```python
from build123d import *

# Parameters (mm, degrees)
SKETCH1_W                    = 38.1
SKETCH1_H                    = 38.1
SKETCH1_W_2                  = 31.75
SKETCH1_H_2                  = 31.75
BOSS_EXTRUDE1_DEPTH          = 238.125
F_10_0_1935_DIAMETER_HOLE2_D = 4.9149


with BuildPart() as part:
    # Sketch1 → Boss-Extrude1 (new body)
    with BuildSketch(Plane.XY):
        Rectangle(SKETCH1_W, SKETCH1_H)
        Rectangle(SKETCH1_W_2, SKETCH1_H_2, mode=Mode.SUBTRACT)
    extrude(amount=BOSS_EXTRUDE1_DEPTH)

    # #10 (0.1935) Diameter Hole2 (through all)
    with Locations(Plane(origin=(0, 19.05, 0), x_dir=(1, 0, 0), z_dir=(0, 1, 0))):
        with Locations((0, -31.75), (0, -89.958333333), (0, -148.166666667), (0, -206.375)):
            Hole(F_10_0_1935_DIAMETER_HOLE2_D / 2)


solid = part.part
```
Verification items for the finished model (mm, model axes). A direction names the side the tool comes from. Give positions to 0.01 mm unless a question says otherwise; leave off trailing zeros. Order: outer loops, then holes, each group sorted by start corner. A loop starts at its lowest first (then second) coordinate and runs counter-clockwise, first axis right, second up. Notation, with made-up numbers: (72, -11) - (79, -11) arc R13 cw to (79, 8) - close; hole circle Ø8 at (8, -25). An arc over 180 degrees is marked (long way). Answer as CSV lines item,"result". Start each with the question number.
Item 1: Mould release check, pull along Z, two halves, no side actions. Record for faces 3 (the face through (0.32, 17.44, 29.313)), 4 (the face through (-15.875, 0, 117)), 5 (the face through (-17, 0, 238.125)), 6 (the face through (0.32, -17.48, 203.94)): released by +Z, released by -Z, zero draft, split by the parting line, or undercut.
Item 2: Section check B-B, the plane x = -11. Record the boundary of the cut face in (y, z) (3 decimals).
Item 3: Access from +Z, -Z, +X, -X, +Y, -Y to the whole of each face (thin tool, end or side, straight path). Record for faces 1 (the face through (0, 19.05, 117)), 2 (the face through (0, 15.875, 117)).
Item 4: Section check A-A, the plane z = 31.75. Record the boundary of the cut face in (x, y) (3 decimals).
Item 5: Section check D-D, the plane x = 0. State how many separate pieces and enclosed holes the cut face has, plus the area to 3 significant figures.
Item 6: Material ranges on L1, parallel to Z at x = 0, y = 18 (3 decimals); L2, parallel to Y at x = 3.5, z = 223.5 (3 decimals), recorded low to high.
Filled in:
1,face 3,"undercut"
1,face 4,"zero draft"
1,face 5,"released by +Z"
1,face 6,"undercut"
2,outline,"(-19.05, 0) - (-15.875, 0) - (-15.875, 238.125) - (-19.05, 238.125) - close; (15.875, 0) - (19.05, 0) - (19.05, 238.125) - (15.875, 238.125) - close"
3,face 1,"+Z, -Z, +X, -X, +Y"
3,face 2,"+Z, -Z"
4,outline,"(-19.05, -19.05) - (-2.457, -19.05) - (-2.457, -15.875) - (-15.875, -15.875) - (-15.875, 15.875) - (-2.457, 15.875) - (-2.457, 19.05) - (-19.05, 19.05) - close; (2.457, -19.05) - (19.05, -19.05) - (19.05, 19.05) - (2.457, 19.05) - (2.457, 15.875) - (15.875, 15.875) - (15.875, -15.875) - (2.457, -15.875) - close"
5,separate pieces,"10"
5,enclosed holes,"0"
5,area,"1,390 mm^2"
6,L1,"0 to 29.293, 34.207 to 87.501, 92.416 to 145.709, 150.624 to 203.918, 208.832 to 238.125"
6,L2,"-19.05 to -15.875, 15.875 to 19.05"
